The model under review builds one solid part; all positions refer to its coordinate system, in mm. A direction names the side the tool comes from. Give positions to 0.01 mm unless a question says otherwise; leave off trailing zeros. Loops run counter-clockwise (first coordinate to the right, second up) from the corner with the lowest first, then second, coordinate; pieces in that order, holes last. Notation, with made-up numbers: (-15.5, 80.5) -> (13.5, 80.5) arc R19 ccw to (13.5, 99.5) -> close; hole circle Ø9 at (88, 72.25). An arc over 180 degrees is marked (long way). Write each question's results on one line, items separated by ' | '. Start each with the question number.
Q1. We need section D-D (z = 31.5). Write out the cut boundary in (x, y), plus the area to 3 significant figures.
Q2. Mouldability with a two-part tool opening along Y and no side actions: class faces 4 (the face through (-20, -2, -10)), 5 (the face through (-44.308, 12.004, -15.863)), 6 (the face through (-22, -21, -2)), 7 (the face through (2, 24, 4)) as released by +Y, released by -Y, zero draft, split by the parting line, or undercut.
Q3. Insertion check: pin 1 Ø12 at (y, z) = (23, 24.5) entering from -X; pin 2 Ø6 at (x, z) = (-24, -18) entering from +Y; pin 3 Ø11.5 at (x, z) = (-34, -9) entering from -Y. Each pin has a flat end and moves straight along its axis. Give the tip position at first contact, or say it passes through.
Q4. We need section C-C (y = 9.5). Write out the cut boundary in (x, z), plus the area to 3 significant figures.
Q5. Wall thickness on L1, parallel to Z at x = 2.9, y = -22.3; L2, parallel to Y at x = 2, z = 36; L3, parallel to Z at x = -18, y = 16: over which ranges is each line inside the solid? List them lowest first. Write a range as [from, to].
Q6. We need section B-B (z = 11.5). Write out the cut boundary in (x, y).
Q7. Machinability: for faces 1 (the face through (0, -20, 24)), 2 (the face through (-44.371, -11.926, -15.907)), 3 (the face through (2, -24, 4)), which of the approach directions +Z, -Z, +X, -X, +Y, -Y give a long, thin tool a straight path to every point of the face, cutting with its end or side? Answer none if there is none.
Q8. We need section A-A (y = -22.3). Write out the cut boundary in (x, z), plus the area to 3 significant figures.
from build123d import *

# Parameters (mm, degrees)
SKETCH1_R           = 16.8
BOSS_EXTRUDE1_DEPTH = 4
BOSS_EXTRUDE2_DEPTH = 40
BOSS_EXTRUDE3_START = 4
BOSS_EXTRUDE3_DEPTH = 40
CUT_EXTRUDE1_REACH  = 58.049
SKETCH4_R           = 1.75
SKETCH6_W           = 20.8
SKETCH6_H           = 42
BOSS_EXTRUDE5_DEPTH = 4
BOSS_EXTRUDE7_REACH = 69.821
SKETCH14_R          = 1.5
CUT_EXTRUDE7_DEPTH  = 62.710359375
CUT_EXTRUDE8_START  = -3
SKETCH15_W          = 27
SKETCH15_H          = 10
SKETCH15_W_2        = 42
CUT_EXTRUDE8_DEPTH  = 59.710359375
SKETCH16_W          = 10
SKETCH16_H          = 23
CUT_EXTRUDE9_DEPTH  = 62.710359375
CUT_EXTRUDE10_DEPTH = 1
FILLET2_R           = 59
FILLET4_R           = 6
BOSS_EXTRUDE8_DEPTH = 25
BOSS_EXTRUDE9_START = -13.299219
SKETCH19_W          = 12
SKETCH19_H          = 2
BOSS_EXTRUDE9_DEPTH = 11.299219


# Read off the part's stored shape, not the designer's step: Boss-Extrude3
with BuildPart() as part:
    # Sketch1 → Boss-Extrude1 (new body)
    with BuildSketch(Plane(origin=(0, 0, 0), x_dir=(0, 1, 0), z_dir=(0, 0, 1))):
        with Locations(Location((0, 0, 0), (0, 0, 270))):
            Circle(SKETCH1_R)
    extrude(amount=BOSS_EXTRUDE1_DEPTH)

    # Sketch2 → Boss-Extrude2 (add)
    with BuildSketch(Plane.XY.offset(4)):
        with BuildLine():
            Line((0, 16.8), (0, 12.8))
            ThreePointArc((0, 12.8), (12.8, 0), (0, -12.8))
            Line((0, -12.8), (0, -16.8))
            ThreePointArc((0, -16.8), (16.8, 0), (0, 16.8))
        make_face()
    extrude(amount=BOSS_EXTRUDE2_DEPTH)

    # Boss-Extrude3 outline → Boss-Extrude3 (add)
    with BuildSketch(Plane.XY.offset(BOSS_EXTRUDE3_START)):
        with BuildLine():
            Line((0, 27.8), (0, 16.8))
            ThreePointArc((0, 16.8), (2.014536045, 16.678778268), (4, 16.316862443))
            Line((4, 16.316862443), (4, 27.8))
            Line((4, 27.8), (0, 27.8))
        make_face()
        with BuildLine():
            ThreePointArc((4, -16.316862443), (2.014536045, -16.678778268), (0, -16.8))
            Line((0, -16.8), (0, -27.8))
            Line((0, -27.8), (4, -27.8))
            Line((4, -27.8), (4, -16.316862443))
        make_face()
    extrude(amount=BOSS_EXTRUDE3_DEPTH)

    # Sketch4 → Cut-Extrude1 (cut, up to next)
    with BuildSketch(Plane.YZ.offset(4), mode=Mode.PRIVATE) as cut_extrude1_sk1:
        with Locations((22.3, 36.5)):
            Circle(SKETCH4_R)
    cut_extrude1_tool1 = extrude(cut_extrude1_sk1.sketch, amount=-CUT_EXTRUDE1_REACH, mode=Mode.PRIVATE) & part.part
    # Sketch4 → Cut-Extrude1 (cut, up to next)
    with BuildSketch(Plane.YZ.offset(4), mode=Mode.PRIVATE) as cut_extrude1_sk2:
        with Locations((22.3, 11.5)):
            Circle(SKETCH4_R)
    cut_extrude1_tool2 = extrude(cut_extrude1_sk2.sketch, amount=-CUT_EXTRUDE1_REACH, mode=Mode.PRIVATE) & part.part
    # Sketch4 → Cut-Extrude1 (cut, up to next)
    with BuildSketch(Plane.YZ.offset(4), mode=Mode.PRIVATE) as cut_extrude1_sk3:
        with Locations((-22.3, 11.5)):
            Circle(SKETCH4_R)
    cut_extrude1_tool3 = extrude(cut_extrude1_sk3.sketch, amount=-CUT_EXTRUDE1_REACH, mode=Mode.PRIVATE) & part.part
    # Sketch4 → Cut-Extrude1 (cut, up to next)
    with BuildSketch(Plane.YZ.offset(4), mode=Mode.PRIVATE) as cut_extrude1_sk4:
        with Locations((-22.3, 36.5)):
            Circle(SKETCH4_R)
    cut_extrude1_tool4 = extrude(cut_extrude1_sk4.sketch, amount=-CUT_EXTRUDE1_REACH, mode=Mode.PRIVATE) & part.part
    add(cut_extrude1_tool1.solids().sort_by_distance((4, 22.3, 36.5))[0], mode=Mode.SUBTRACT)
    add(cut_extrude1_tool2.solids().sort_by_distance((4, 22.3, 11.5))[0], mode=Mode.SUBTRACT)
    add(cut_extrude1_tool3.solids().sort_by_distance((4, -22.3, 11.5))[0], mode=Mode.SUBTRACT)
    add(cut_extrude1_tool4.solids().sort_by_distance((4, -22.3, 36.5))[0], mode=Mode.SUBTRACT)

    # Sketch6 → Boss-Extrude5 (add)
    with BuildSketch(Plane(origin=(0, 0, 0), x_dir=(1, 0, 0), z_dir=(0, 0, -1))):
        with Locations((-6.4, 0)):
            Rectangle(SKETCH6_W, SKETCH6_H)
    extrude(amount=-BOSS_EXTRUDE5_DEPTH)

    # Boss-Extrude7: up to this face of the body (flat: up to its plane)
    boss_extrude7_end = Plane(part.part.faces().sort_by_distance((-6.4, -21, 2))[0])
    # Sketch10 → Boss-Extrude7 (add, up to the picked face)
    with BuildSketch(Plane(origin=(0, 21, 0), x_dir=(-1, 0, 0), z_dir=(0, 1, 0)), mode=Mode.PRIVATE) as boss_extrude7_sk1:
        Polygon((-4, 0), (49.483656551, -22.54766646), (51.20438586, -20.090210327), (16.8, 4), (-4, 4), align=None)
    boss_extrude7_tool1 = split(extrude(boss_extrude7_sk1.sketch, amount=-BOSS_EXTRUDE7_REACH, mode=Mode.PRIVATE), bisect_by=boss_extrude7_end, keep=Keep.BOTH, mode=Mode.PRIVATE)
    add(boss_extrude7_tool1.solids().sort_by(Axis((-21.697526, 21, -6.303092), (0, -1, 0)))[0])

    # Sketch14 → Cut-Extrude7 (cut, through all)
    with BuildSketch(Plane(origin=(-7.406416038, 0, 10.577458301), x_dir=(0.8191520442889908, 0, 0.5735764363510476), z_dir=(-0.5735764363510476, 0, 0.8191520442889909))):
        with Locations((-47.467448599, 14)):
            Circle(SKETCH14_R)
        with Locations((-19.467448599, 14)):
            Circle(SKETCH14_R)
        with Locations(Location((-19.467448599, -14, 0), (0, 0, 180))):
            Circle(SKETCH14_R)
        with Locations(Location((-47.467448599, -14, 0), (0, 0, 180))):
            Circle(SKETCH14_R)
    extrude(amount=-CUT_EXTRUDE7_DEPTH, mode=Mode.SUBTRACT)

    # Sketch15 → Cut-Extrude8 (cut, through all)
    with BuildSketch(Plane(origin=(-7.406416038, 0, 10.577458301), x_dir=(0.8191520442889908, 0, 0.5735764363510476), z_dir=(-0.5735764363510476, 0, 0.8191520442889909)).offset(CUT_EXTRUDE8_START)):
        with Locations((-39.967448599, 16)):
            Rectangle(SKETCH15_W, SKETCH15_H)
        with Locations((-32.467448599, -16)):
            Rectangle(SKETCH15_W_2, SKETCH15_H)
    extrude(amount=-CUT_EXTRUDE8_DEPTH, mode=Mode.SUBTRACT)

    # Sketch16 → Cut-Extrude9 (cut, through all)
    with BuildSketch(Plane(origin=(-7.406416038, 0, 10.577458301), x_dir=(0.8191520442889908, 0, 0.5735764363510476), z_dir=(-0.5735764363510476, 0, 0.8191520442889909))):
        with Locations((-21.967448599, 9.5)):
            Rectangle(SKETCH16_W, SKETCH16_H)
    extrude(amount=-CUT_EXTRUDE9_DEPTH, mode=Mode.SUBTRACT)

    # Sketch17 → Cut-Extrude10 (cut)
    with BuildSketch(Plane(origin=(-7.406416038, 0, 10.577458301), x_dir=(0.8191520442889908, 0, 0.5735764363510476), z_dir=(-0.5735764363510476, 0, 0.8191520442889909))):
        with BuildLine():
            Line((-48.967448599, 10.5), (-48.967448599, -10.5))
            ThreePointArc((-48.967448599, -10.5), (-45.431914693, -11.964466094), (-43.967448599, -15.5))
            Line((-43.967448599, -15.5), (-22.967448599, -15.5))
            ThreePointArc((-22.967448599, -15.5), (-22.539929967, -13.477028389), (-21.330482943, -11.8))
            Line((-21.330482943, -11.8), (-17.967448599, -11.8))
            Line((-17.967448599, -11.8), (-17.967448599, 15.5))
            Line((-17.967448599, 15.5), (-43.967448599, 15.5))
            ThreePointArc((-43.967448599, 15.5), (-45.431914693, 11.964466094), (-48.967448599, 10.5))
        make_face()
    extrude(amount=-CUT_EXTRUDE10_DEPTH, mode=Mode.SUBTRACT)

    # Fillet2
    fillet2_edges = [part.edges().sort_by_distance(p)[0] for p in [
        (4, 0, 0),
    ]]
    fillet(fillet2_edges, radius=FILLET2_R)

    # Fillet4
    fillet4_edges = [part.edges().sort_by_distance(p)[0] for p in [
        (4, 18.658431222, 0),
        (4, -18.658431222, 0),
    ]]
    fillet(fillet4_edges, radius=FILLET4_R)

    # Sketch18 → Boss-Extrude8 (add)
    with BuildSketch(Plane(origin=(0, 21, 0), x_dir=(-1, 0, 0), z_dir=(0, 1, 0))):
        Polygon((28.92328025, -5.709586808), (18.025327959, -21.273475649), (9.833807517, -15.537711286), (8.686654644, -17.176015374), (18.516479175, -24.058932611), (30.561584339, -6.85673968), align=None)
    extrude(amount=-BOSS_EXTRUDE8_DEPTH)

    # Sketch19 → Boss-Extrude9 (add)
    with BuildSketch(Plane(origin=(5.212265562, 0, -7.443886673), x_dir=(0.819152044288991, 0, 0.5735764363510472), z_dir=(0.5735764363510472, 0, -0.819152044288991)).offset(BOSS_EXTRUDE9_START)):
        with Locations((-22.967448599, 3)):
            Rectangle(SKETCH19_W, SKETCH19_H)
    extrude(amount=BOSS_EXTRUDE9_DEPTH)


solid = part.part
Output:
1) outline: (0, -27.8) -> (4, -27.8) -> (4, -16.32) arc R16.8 ccw to (4, 16.32) -> (4, 27.8) -> (0, 27.8) -> (0, 12.8) arc R12.8 cw to (0, -12.8) -> close | area: 275 mm2
2) face 4: released by +Y | face 5: undercut | face 6: released by -Y | face 7: zero draft
3) pin 1: x = 0 | pin 2: y = 21 | pin 3: y = -21
4) outline: (-51.2, -20.09) -> (-49.48, -22.55) -> (-26.39, -12.81) -> (-18.52, -24.06) -> (-8.69, -17.18) -> (-9.83, -15.54) -> (-18.03, -21.27) -> (-28.92, -5.71) -> (-46.94, -18.33) -> (-47.52, -17.51) -> close; (-21.31, 0.85) -> (-15.08, -8.04) -> (-6.99, -4.63) arc R59 cw to (13.86, -0.04) -> (13.86, 44) -> (8.58, 44) -> (8.58, 4) -> (-16.8, 4) -> close | area: 633 mm2
5) L1: [4, 9.75], [13.25, 34.75], [38.25, 44] | L2: [-27.8, -23.98], [-20.62, -12.64], [12.64, 20.62], [23.98, 27.8] | L3: [-23.7, -21.26], [-3.88, 3.16]
6) outline: (0, -27.8) -> (4, -27.8) -> (4, -24.05) -> (0, -24.05) -> close; (0, -20.55) -> (4, -20.55) -> (4, -16.32) arc R16.8 ccw to (4, 16.32) -> (4, 20.55) -> (0, 20.55) -> (0, 12.8) arc R12.8 cw to (0, -12.8) -> close; (0, 24.05) -> (4, 24.05) -> (4, 27.8) -> (0, 27.8) -> close
7) face 1: +Z, -X, +Y, -Y | face 2: +Z | face 3: -Z, +X, -X, -Y
8) outline: (0, 4) -> (4, 4) -> (4, 9.75) -> (0, 9.75) -> close; (0, 13.25) -> (4, 13.25) -> (4, 34.75) -> (0, 34.75) -> close; (0, 38.25) -> (4, 38.25) -> (4, 44) -> (0, 44) -> close | area: 132 mm2
